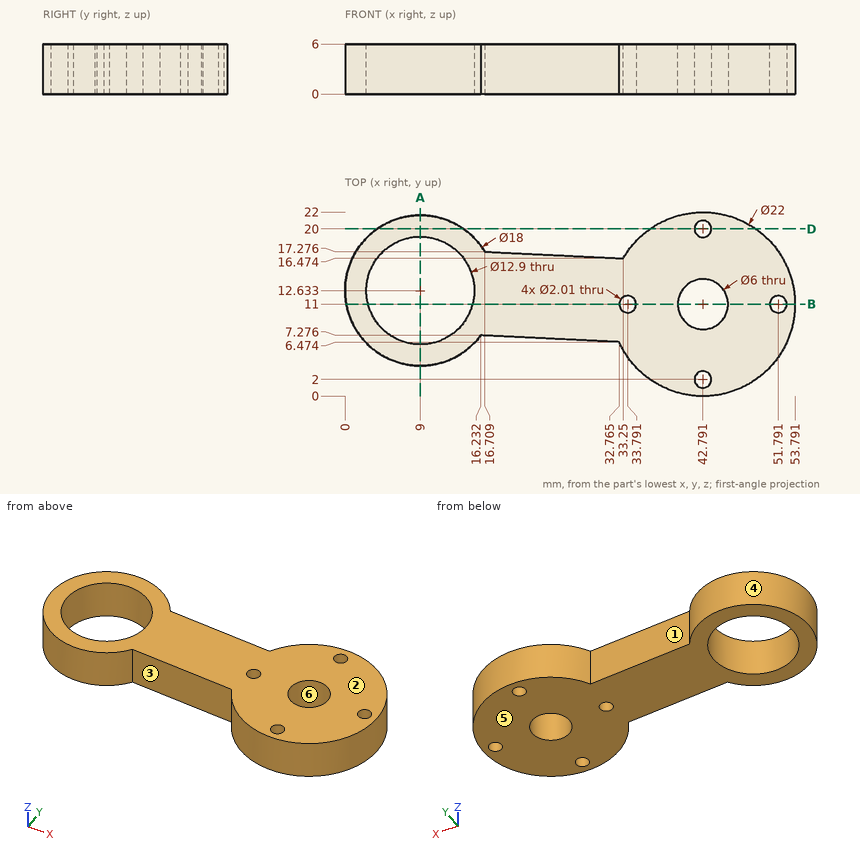
The figure shows three views and two pictorial views of one solid part (mm, origin at its lowest corner). Answer the questions. A direction names the side the tool comes from. Give positions to 0.01 mm unless a question says otherwise; leave off trailing zeros. Order: outer loops, then holes, each group sorted by start corner. A loop starts at its lowest first (then second) coordinate and runs counter-clockwise, first axis right, second up. Notation, with made-up numbers: (48.25, 48) -> (90.25, 48) arc R35 ccw to (90.25, 82) -> close; hole circle Ø10 at (10.5, -16). An arc over 180 degrees is marked (long way). Answer as a JSON object with one key per item and string values. Group by question number.
Item 1: Consider L1, parallel to Y at x = 9, z = 3.45; L2, parallel to X at y = 19.5, z = 2.15 (1 decimal); L3, parallel to X at y = 17.5, z = 5 (1 decimal). Determine where each line is inside the solid, lowest interval first. Write a range as from..to.
Item 2: The part is cut by section B-B on y = 11. Give the number of separate pieces and of enclosed holes in the cut face, and give its area (3 significant figures).
Item 3: The part is cut by section A-A on x = 9. Write down the section's boundary in (y, z).
Item 4: Flat-ended cylindrical pins translate along their axes: pin 1 (3 mm diameter, centred on y = 7, z = 1.5, fed in from +X); pin 2 (1 mm diameter, centred on y = 16, z = 1, fed in from -X); pin 3 (2 mm diameter, centred on y = 10.5, z = 1.5, fed in from -X). Find the tip coordinate at first contact, or state that the pin passes through.
Item 5: Determine the mould class of the marked faces 4, 5 and 6 for opening direction Y: pulls with the +Y half, pulls with the -Y half, needs draft (parallel to the pull), parting line crosses it, or undercut.
Item 6: The part is cut by section D-D on y = 20. Write down the section's boundary in (x, z) (1 decimal), and give its area (3 significant figures).
Item 7: A tool of negligible diameter and unlimited length cuts with its end or side. For the marked faces 1, 2 and 3, from which of +Z, -Z, +X, -X, +Y, -Y can it reach the whole face along a straight path? Write none if from no direction.
Result set:
{
 "1": {"L1": "3.63..6.18, 19.08..21.63", "L2": "3.2..14.8, 35.8..41.9, 43.7..49.8", "L3": "1.4..4.8, 13.2..16.6, 33.9..51.7"},
 "2": {"separate pieces": "5", "enclosed holes": "0", "area": "187 mm²"},
 "3": {"outline": "(3.63, 0) -> (6.18, 0) -> (6.18, 6) -> (3.63, 6) -> close; (19.08, 0) -> (21.63, 0) -> (21.63, 6) -> (19.08, 6) -> close"},
 "4": {"pin 1": "x = 53.5", "pin 2": "x = 0.47", "pin 3": "x = 0.07"},
 "5": {"face 4": "parting line crosses it", "face 5": "needs draft", "face 6": "undercut"},
 "6": {"outline": "(3.8, 0) -> (14.2, 0) -> (14.2, 6) -> (3.8, 6) -> close; (36.5, 0) -> (41.8, 0) -> (41.8, 6) -> (36.5, 6) -> close; (43.8, 0) -> (49.1, 0) -> (49.1, 6) -> (43.8, 6) -> close", "area": "126 mm²"},
 "7": {"face 1": "+Z, -Z, +Y", "face 2": "+Z, +X, -X, +Y, -Y", "face 3": "+Z, -Z, -Y"}
}
